Work out the finished part from the listing and answer in its coordinate system (mm). Give positions to 0.01 mm unless a question says otherwise; leave off trailing zeros. Loops run counter-clockwise (first coordinate to the right, second up) from the corner with the lowest first, then second, coordinate; pieces in that order, holes last. Notation, with made-up numbers: (9.5, 47.5) -> (51.5, 47.5) arc R24 ccw to (51.5, 69.5) -> close; hole circle Ø3 at (-32, 75.5). An arc over 180 degrees is marked (long way). Answer as CSV lines item,"result". Start each with the question number.
1. A flat-ended cylindrical pin translates along its axis: pin 1 Ø1.9 at (x, z) = (-812.5, 3) entering from -Y. Find the tip coordinate at first contact, or state that the pin passes through.
2. Find the intervals of material crossed by line 1 along X through (y, z) = (293.5, 1.75); line 2 along X through (y, z) = (170.5, 6); line 3 along Y through (x, z) = (-933, 6), in increasing order.
3. Find section A-A, the plane y = 304.5. Give the vertices of the cut face in (x, z).
4. Find section B-B, the plane z = 2.5. Count the separate pieces of the cut face and the enclosed holes in it, and give its area (3 significant figures).
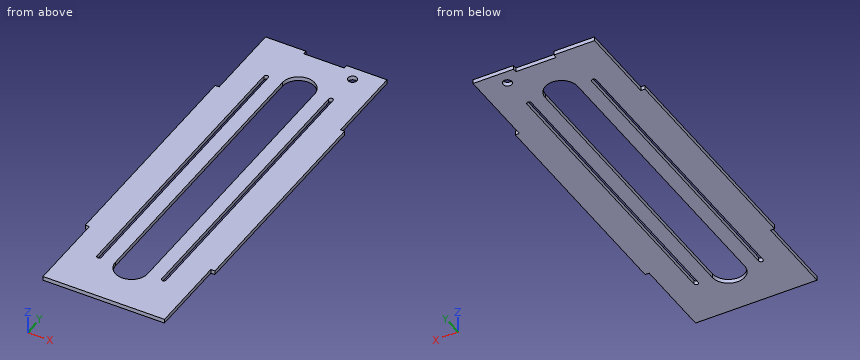
from build123d import *

# Parameters (mm, degrees)
SKETCH2_W                = 215.9
SKETCH2_H                = 609.6
BOSS_EXTRUDE1_DEPTH      = 6.35
CUT_EXTRUDE1_DEPTH       = 7.35
CUT_EXTRUDE2_DEPTH       = 1
CUT_EXTRUDE2_DEPTH_BACK  = 7.35
CUT_EXTRUDE3_DEPTH       = 1
CUT_EXTRUDE3_DEPTH_BACK  = 7.35
CUT_EXTRUDE6_DEPTH       = 1
CUT_EXTRUDE6_DEPTH_BACK  = 7.35
CUT_EXTRUDE7_DEPTH       = 1
CUT_EXTRUDE7_DEPTH_BACK  = 7.35
CUT_EXTRUDE11_DEPTH      = 1
CUT_EXTRUDE11_DEPTH_BACK = 7.35
CUT_EXTRUDE13_DEPTH      = 1
CUT_EXTRUDE13_DEPTH_BACK = 7.35
SKETCH13_W               = 63.5
SKETCH13_H               = 6.35
CUT_EXTRUDE14_DEPTH      = 1
CUT_EXTRUDE14_DEPTH_BACK = 7.35
CUT_EXTRUDE19_DEPTH      = 7.35
SKETCH26_R               = 6.985
CUT_EXTRUDE20_DEPTH      = 7.35


with BuildPart() as part:
    # Sketch2 → Boss-Extrude1 (new body)
    with BuildSketch(Plane.XY):
        with Locations((-911.126767395, 370.108550968)):
            Rectangle(SKETCH2_W, SKETCH2_H)
    extrude(amount=BOSS_EXTRUDE1_DEPTH)

    # Sketch3 → Cut-Extrude1 (cut, through all)
    with BuildSketch(Plane.XY.offset(6.35)):
        with BuildLine():
            Line((-936.526767395, 141.508550968), (-936.526767395, 598.708550968))
            ThreePointArc((-936.526767395, 598.708550968), (-911.126767395, 624.108550968), (-885.726767395, 598.708550968))
            Line((-885.726767395, 598.708550968), (-885.726767395, 141.508550968))
            ThreePointArc((-885.726767395, 141.508550968), (-911.126767395, 116.108550968), (-936.526767395, 141.508550968))
        make_face()
    extrude(amount=-CUT_EXTRUDE1_DEPTH, mode=Mode.SUBTRACT)

    # Sketch4 → Cut-Extrude2 (cut, two sides)
    with BuildSketch(Plane.XY.offset(6.35)) as cut_extrude2_sk:
        Polygon((-815.876767395, 1970.05819206), (-815.876767395, 674.908550968), (-815.876767395, 547.908550968), (-803.176767395, 547.908550968), (491.972873698, 547.908550968), (2398.607136056, 2301.304159748), (1090.757494964, 3723.45380084), align=None)
    extrude(amount=CUT_EXTRUDE2_DEPTH, mode=Mode.SUBTRACT)
    extrude(cut_extrude2_sk.sketch, amount=-CUT_EXTRUDE2_DEPTH_BACK, mode=Mode.SUBTRACT)

    # Sketch5 → Cut-Extrude3 (cut, two sides)
    with BuildSketch(Plane.XY.offset(6.35)) as cut_extrude3_sk:
        Polygon((-815.876767395, -1229.841090125), (-815.876767395, 65.308550968), (-815.876767395, 192.308550968), (-803.176767395, 192.308550968), (491.972873698, 192.308550968), (2398.607136056, -1561.087057812), (1090.757494964, -2983.236698905), align=None)
    extrude(amount=CUT_EXTRUDE3_DEPTH, mode=Mode.SUBTRACT)
    extrude(cut_extrude3_sk.sketch, amount=-CUT_EXTRUDE3_DEPTH_BACK, mode=Mode.SUBTRACT)

    # Sketch6 → Cut-Extrude6 (cut, two sides)
    with BuildSketch(Plane.XY.offset(6.35)) as cut_extrude6_sk:
        Polygon((-1006.376767395, 1970.05819206), (-1006.376767395, 674.908550968), (-1006.376767395, 547.908550968), (-1019.076767395, 547.908550968), (-2314.226408487, 547.908550968), (-4220.860670845, 2301.304159748), (-2913.011029753, 3723.45380084), align=None)
    extrude(amount=CUT_EXTRUDE6_DEPTH, mode=Mode.SUBTRACT)
    extrude(cut_extrude6_sk.sketch, amount=-CUT_EXTRUDE6_DEPTH_BACK, mode=Mode.SUBTRACT)

    # Sketch9 → Cut-Extrude7 (cut, two sides)
    with BuildSketch(Plane.XY.offset(6.35)) as cut_extrude7_sk:
        Polygon((-1006.376767395, -1229.841090125), (-1006.376767395, 65.308550968), (-1006.376767395, 192.308550968), (-1019.076767395, 192.308550968), (-2314.226408487, 192.308550968), (-4220.860670845, -1561.087057812), (-2913.011029753, -2983.236698905), align=None)
    extrude(amount=CUT_EXTRUDE7_DEPTH, mode=Mode.SUBTRACT)
    extrude(cut_extrude7_sk.sketch, amount=-CUT_EXTRUDE7_DEPTH_BACK, mode=Mode.SUBTRACT)

    # Sketch16 → Cut-Extrude11 (cut, two sides)
    with BuildSketch(Plane.XY.offset(6.35)) as cut_extrude11_sk:
        Polygon((-1012.726767395, -869.953702465), (-1012.726767395, 192.308550968), (-1012.726767395, 547.908550968), (-1012.726767395, 1610.170804401), (-3137.251274261, 1610.170804401), (-3137.251274261, -869.953702465), align=None)
    extrude(amount=CUT_EXTRUDE11_DEPTH, mode=Mode.SUBTRACT)
    extrude(cut_extrude11_sk.sketch, amount=-CUT_EXTRUDE11_DEPTH_BACK, mode=Mode.SUBTRACT)

    # Sketch17 → Cut-Extrude13 (cut, two sides)
    with BuildSketch(Plane.XY.offset(6.35)) as cut_extrude13_sk:
        Polygon((-809.526767395, -864.960277939), (-809.526767395, 192.308550968), (-809.526767395, 547.908550968), (-809.526767395, 1605.177379875), (1305.010890419, 1605.177379875), (1305.010890419, -864.960277939), align=None)
    extrude(amount=CUT_EXTRUDE13_DEPTH, mode=Mode.SUBTRACT)
    extrude(cut_extrude13_sk.sketch, amount=-CUT_EXTRUDE13_DEPTH_BACK, mode=Mode.SUBTRACT)

    # Sketch13 → Cut-Extrude14 (cut, two sides)
    with BuildSketch(Plane(origin=(0, 0, 0), x_dir=(-1, 0, 0), z_dir=(0, 0, -1))) as cut_extrude14_sk:
        with Locations((911.126767395, 671.733550968)):
            Rectangle(SKETCH13_W, SKETCH13_H)
    extrude(amount=CUT_EXTRUDE14_DEPTH, mode=Mode.SUBTRACT)
    extrude(cut_extrude14_sk.sketch, amount=-CUT_EXTRUDE14_DEPTH_BACK, mode=Mode.SUBTRACT)

    # Sketch25 → Cut-Extrude19 (cut, through all)
    with BuildSketch(Plane(origin=(0, 0, 0), x_dir=(-1, 0, 0), z_dir=(0, 0, -1))):
        with BuildLine():
            Line((958.497767395, 141.508550968), (958.497767395, 598.708550968))
            ThreePointArc((958.497767395, 598.708550968), (961.926767395, 602.137550968), (965.355767395, 598.708550968))
            Line((965.355767395, 598.708550968), (965.355767395, 141.508550968))
            ThreePointArc((965.355767395, 141.508550968), (961.926767395, 138.079550968), (958.497767395, 141.508550968))
        make_face()
    cut_extrude19 = extrude(amount=-CUT_EXTRUDE19_DEPTH, mode=Mode.SUBTRACT)

    # Mirror1: Cut-Extrude19 across plane
    add(cut_extrude19.mirror(Plane(origin=(-911.126767395, 0, 0), x_dir=(0, 0, 1), z_dir=(1, 0, 0))), mode=Mode.SUBTRACT)

    # Sketch26 → Cut-Extrude20 (cut, through all)
    with BuildSketch(Plane.XY.offset(6.35)):
        with Locations((-857.158491521, 652.784891731)):
            Circle(SKETCH26_R)
    extrude(amount=-CUT_EXTRUDE20_DEPTH, mode=Mode.SUBTRACT)


solid = part.part
Resolved:
1,pin 1,"stops at y = 192.31"
2,line 1,"x = -1012.73 to -965.36, -958.5 to -936.53, -885.73 to -863.76, -856.9 to -809.53"
2,line 2,"x = -1006.38 to -965.36, -958.5 to -936.53, -885.73 to -863.76, -856.9 to -815.88"
2,line 3,"y = 65.31 to 128.6, 611.62 to 668.56"
3,outline,"(-1012.73, 0) -> (-965.36, 0) -> (-965.36, 6.35) -> (-1012.73, 6.35) -> close; (-958.5, 0) -> (-936.53, 0) -> (-936.53, 6.35) -> (-958.5, 6.35) -> close; (-885.73, 0) -> (-863.76, 0) -> (-863.76, 6.35) -> (-885.73, 6.35) -> close; (-856.9, 0) -> (-809.53, 0) -> (-809.53, 6.35) -> (-856.9, 6.35) -> close"
4,separate pieces,"1"
4,enclosed holes,"4"
4,area,"88,500 mm^2"
